Check sheet for the modelled part. Datum: model origin and axes. Units: mm. Round coordinates to 2 decimals unless told otherwise and drop trailing zeros. Loops run counter-clockwise (first coordinate to the right, second up) from the corner with the lowest first, then second, coordinate; pieces in that order, holes last. Notation, with made-up numbers: M -33.5,34 L -2.5,34 A28 cw -2.5,72 Z; hole C 72,65 d1. An arc over 180 degrees is marked long. One line per question, with ' | ' between items. Start each with the question number.
(1) Section check B-B (z = -23). Record the boundary of the cut face in (x, y).
(2) Thickness scan on probe 1 along X at (y, z) = (126.75, -43.5); probe 2 along Y at (x, z) = (1, -24); probe 3 along Y at (x, z) = (26.5, -48). Record the ranges inside material, lowest first. Write a range as [from, to].
(3) Go/stop test with flat-tipped pins: P1, Ø3, axis at x = -16, z = -50, coming from the -Y side; P2, Ø4, axis at x = -19.5, z = -25.5, coming from the -Y side; P3, Ø6, axis at y = 130, z = -30.5, coming from the +X side. Record where each tip stops, or that it passes through.
(4) Section check D-D (y = 131). Record the boundary of the cut face in (x, z).
(5) Section check A-A (y = 119). Record the boundary of the cut face in (x, z).
(6) Section check C-C (x = -14). Record the boundary of the cut face in (y, z), and give its area (3 significant figures).
(7) Draft check along X on faces 1 (the face through (-0.4, 120.5, -37.6)), 2 (the face through (0, 125, -17.305)), 3 (the face through (33.576, 127.55, -37.025)). Enter one of: +X half, -X half, draft (parallel to the pull), parting line (faces both ways), or undercut.
Autodesk Inventor part; units mm, degrees
ref_plane "РабПлоскость2" through (-132.2012, -132.5, -3) normal (0, 0, -1) x (0, 1, 0)
ref_plane "YZ Plane" through (0, 0, 0) normal (1, 0, 0) x (0, 1, 0)
ref_plane "XZ Plane" through (0, 0, 0) normal (0, 1, 0) x (-1, 0, 0)
ref_plane "РабПлоскость1" through (0, 0, -57.3048) normal (0, 0, 1) x (-1, 0, 0)
sketch "Эскиз1" plane through (0, 0, -57.3048) normal (0, 0, 1) x (-1, 0, 0)
  circle A0 centre (0, 0) radius 132.5
  line L0 (31.1877, -116.3941) -> (34.2935, -127.9852)
  arc A1 (-31.1877, -116.3941) -> (31.1877, -116.3941) centre (0, 0) ccw
  line L1 (-34.2935, -127.9852) -> (-31.1877, -116.3941)
  point P0 (0, 0)
ref_plane "РабПлоскость2" through (-132.2012, -132.5, -3) normal (0, 0, -1) x (0, 1, 0)
extrude "Выдавливание1" add sketch "Эскиз1" along normal blind 40 contours L1 A1 L0 A0 picked at (24.6238, -125.9568)
fillet "Сопряжение1" radius 2 4 edges at (34.2935, 127.9852, -37.3048) (31.1877, 116.3941, -37.3048) (-31.1877, 116.3941, -37.3048) (-34.2935, 127.9852, -37.3048)
properties part number "Стойка"
The answers:
1) outline: M -33.77,126.04 L -31.7,118.31 A2 ccw -29.28,116.89 A120.5 cw 29.28,116.89 A2 ccw 31.7,118.31 L 33.77,126.04 A2 ccw 32.33,128.5 A132.5 ccw -32.33,128.5 A2 ccw Z
2) probe 1: [-33.83, 33.83] | probe 2: [120.5, 132.5] | probe 3: [117.55, 129.82]
3) P1: y = 119.22 | P2: y = 118.57 | P3: x = 33.79
4) outline: M -19.88,-57.3 L 19.88,-57.3 L 19.88,-17.3 L -19.88,-17.3 Z
5) outline: M -31.89,-57.3 L -18.95,-57.3 L -18.95,-17.3 L -31.89,-17.3 Z; M 18.95,-57.3 L 31.89,-57.3 L 31.89,-17.3 L 18.95,-17.3 Z
6) outline: M 119.68,-57.3 L 131.76,-57.3 L 131.76,-17.3 L 119.68,-17.3 Z | area: 483 mm²
7) face 1: undercut | face 2: draft | face 3: +X half
